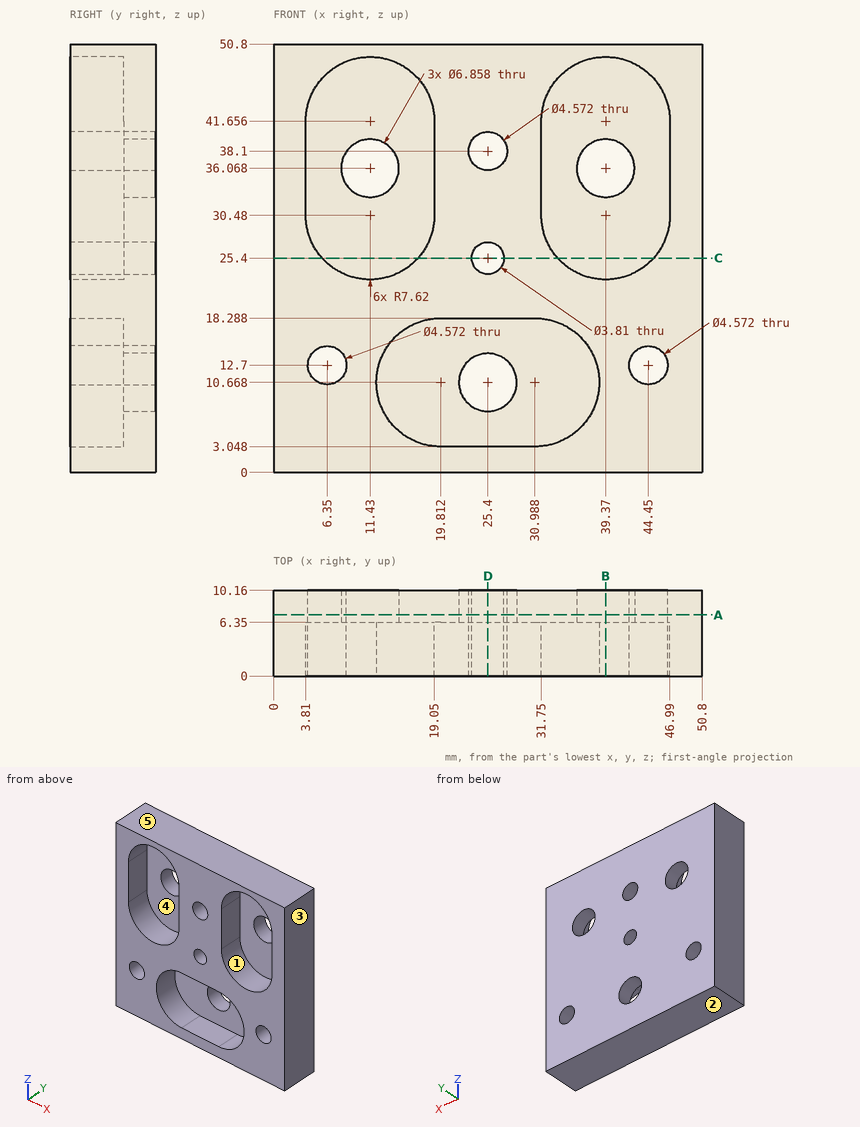
The drawing under review shows one solid part. Ordinate dimensions are in mm from its lowest x, y, z. A direction names the side the tool comes from. Round coordinates to 2 decimals unless told otherwise and drop trailing zeros. Loops run counter-clockwise (first coordinate to the right, second up) from the corner with the lowest first, then second, coordinate; pieces in that order, holes last. Notation, with made-up numbers: (18.25, 12.5) - (49.25, 12.5) arc R20 ccw to (49.25, 33.5) - close; hole circle Ø10 at (47, -4). An arc over 180 degrees is marked (long way). One line per item, written item: value. Start each with the question number.
1) To check wall thickness, follow L1, parallel to X at y = 3.25, z = 38; L2, parallel to Z at x = 30, y = 4; L3, parallel to Z at x = 45, y = 5.5. State the ranges of each line that lie inside material, in increasing order. Write a range as from..to.
2) For the marked faces 4 and 5, list the 3-axis set-ups (+Z, -Z, +X, -X, +Y, -Y) from which the entire face can be reached by the end or side of a thin tool; tool diameter is ignored.
3) Consider section C-C on z = 25.4. Give the boundary of the cut face in (x, y) (3 decimals).
4) Consider section B-B on x = 39.37. Give the boundary of the cut face in (y, z), then the cut area to 3 significant figures.
5) Consider section D-D on x = 25.4. Give the boundary of the cut face in (y, z) (3 decimals), then the cut area to 3 significant figures.
6) Consider section A-A on y = 7.25. Give the boundary of the cut face in (x, z) (3 decimals), then the cut area to 3 significant figures.
7) Draft analysis for pull direction Z (two halves, no side actions). For the marked faces 1, 2 and 3, state which applies: +Z half, -Z half, draft (parallel to the pull), parting line (faces both ways), or undercut.
8) Insertion check: pin 1 Ø3 at (x, z) = (25.4, 25.4) entering from +Y; pin 2 Ø9 at (x, z) = (39.37, 36.068) entering from -Y. Each pin has a flat end and moves straight along its axis. Give the tip position at first contact, or say it passes through.
Reported:
1. L1: x = 0..3.81, 19.05..23.12, 27.68..31.75, 46.99..50.8
1. L2: z = 0..3.05, 18.29..50.8
1. L3: z = 0..10.48, 14.92..25.35, 46.79..50.8
2. face 4: -Y
2. face 5: +Z, +X, -X, +Y, -Y
3. outline: (0, 0) - (5.75, 0) - (5.75, 6.35) - (17.11, 6.35) - (17.11, 0) - (23.495, 0) - (23.495, 10.16) - (0, 10.16) - close; (27.305, 0) - (33.69, 0) - (33.69, 6.35) - (45.05, 6.35) - (45.05, 0) - (50.8, 0) - (50.8, 10.16) - (27.305, 10.16) - close
4. outline: (0, 0) - (10.16, 0) - (10.16, 32.64) - (6.35, 32.64) - (6.35, 22.86) - (0, 22.86) - close; (0, 49.28) - (6.35, 49.28) - (6.35, 39.5) - (10.16, 39.5) - (10.16, 50.8) - (0, 50.8) - close
4. area: 322 mm^2
5. outline: (0, 0) - (10.16, 0) - (10.16, 7.239) - (6.35, 7.239) - (6.35, 3.048) - (0, 3.048) - close; (0, 18.288) - (6.35, 18.288) - (6.35, 14.097) - (10.16, 14.097) - (10.16, 23.495) - (0, 23.495) - close; (0, 27.305) - (10.16, 27.305) - (10.16, 35.814) - (0, 35.814) - close; (0, 40.386) - (10.16, 40.386) - (10.16, 50.8) - (0, 50.8) - close
5. area: 308 mm^2
6. outline: (0, 0) - (50.8, 0) - (50.8, 50.8) - (0, 50.8) - close; hole circle Ø4.572 at (6.35, 12.7); hole circle Ø6.858 at (11.43, 36.068); hole circle Ø6.858 at (25.4, 10.668); hole circle Ø4.572 at (25.4, 38.1); hole circle Ø3.81 at (25.4, 25.4); hole circle Ø6.858 at (39.37, 36.068); hole circle Ø4.572 at (44.45, 12.7)
6. area: 2,410 mm^2
7. face 1: undercut
7. face 2: -Z half
7. face 3: draft
8. pin 1: passes through
8. pin 2: stops at y = 6.35
